CAD build for the part. Positions are in the model's coordinates, mm. Round coordinates to 2 decimals unless told otherwise and drop trailing zeros. Loops run counter-clockwise (first coordinate to the right, second up) from the corner with the lowest first, then second, coordinate; pieces in that order, holes last.
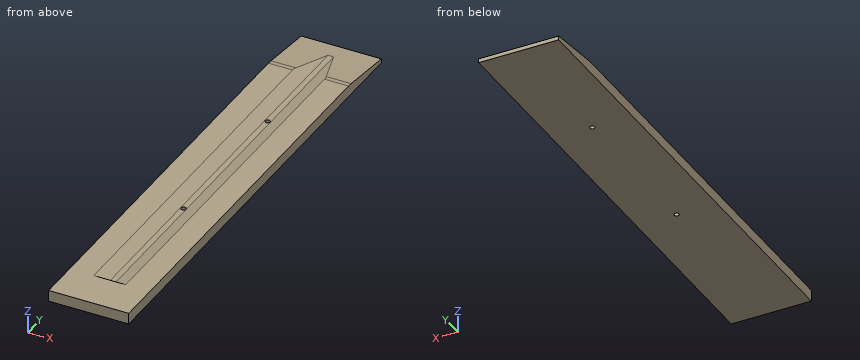
```python
from build123d import *

# Parameters (mm, degrees)
F1_DEPTH = 20
F3_DEPTH = 120
F6_R     = 0.6
F7_DEPTH = 25
F8_R     = 10


with BuildPart() as f1:
    # F0 (on Right) → F1 (new body)
    with BuildSketch(Plane.YZ):
        Polygon((0, 2.8), (0, 0), (120, 0), (120, 1), (105, 2.8), align=None)
    extrude(amount=F1_DEPTH)


with BuildPart() as f3:
    # F2 (on face) → F3 (new body)
    with BuildSketch(Plane.XZ):
        Polygon((6, 2.8), (9.296973, 1.6), (10.703027, 1.6), (14, 2.8), align=None)
    extrude(amount=-F3_DEPTH)


with BuildPart() as f3_1:
    # F4: moved
    add(f3.part.moved(Location((0, 10, 0))))


with BuildPart() as f1_1:
    add(f1.part)

    # F5: cut F3
    add(f3_1.part, mode=Mode.SUBTRACT)

    # F6 (on face) → F7 (cut)
    with BuildSketch(Plane.XY.offset(1.6)):
        with Locations((10, 85)):
            Circle(F6_R)
        with Locations((10, 45)):
            Circle(F6_R)
    extrude(amount=-F7_DEPTH, mode=Mode.SUBTRACT)

    # F8
    f8_edges = [f1_1.edges().sort_by_distance(p)[0] for p in [
        (17, 105, 2.8),
        (3, 105, 2.8),
    ]]
    fillet(f8_edges, radius=F8_R)


solid = f1_1.part
```
Item 1: Probe line 1 (Y direction, x = 10, z = 0.4); line 2 (X direction, y = 85, z = 1); line 3 (Z direction, x = 10.25, y = 96.5). List the from-to ranges inside material, lowest first.
Answers follow:
line 1: y = 0 to 44.4, 45.6 to 84.4, 85.6 to 120
line 2: x = 0 to 9.4, 10.6 to 20
line 3: z = 0 to 1.6
Item 2: Cut at C-C, the plane z = 2.15. Give the cut face in (x, y), plus the area to 3 significant figures.
Answers follow:
outline: (0, 0) - (20, 0) - (20, 110.42) - (12.21, 110.42) - (12.21, 10) - (7.79, 10) - (7.79, 110.42) - (0, 110.42) - close
area: 1,760 mm2
Item 3: Cut at A-A, the plane y = 94. Give the cut face in (x, z), plus the area to 3 significant figures.
Answers follow:
outline: (0, 0) - (20, 0) - (20, 2.8) - (14, 2.8) - (10.7, 1.6) - (9.3, 1.6) - (6, 2.8) - (0, 2.8) - close
area: 50.4 mm2
Item 4: Cut at B-B, the plane x = 15.5. Give the cut face in (y, z).
Answers follow:
outline: (0, 0) - (120, 0) - (120, 1) - (105.59, 2.73) arc R10 ccw to (104.4, 2.8) - (0, 2.8) - close
Item 5: Flat gauge pins, fed straight in: P1, Ø1.5, axis at x = 10.5, y = 46.5, coming from the +Z side; P2, Ø12, axis at x = 14, y = 100, coming from the -Z side. Where does each tip first touch, or does it go through?
Answers follow:
P1: stops at z = 1.8
P2: stops at z = 0
Item 6: Cut at D-D, the plane x = 8.25. Give the cut face in (y, z), plus the area to 3 significant figures.
Answers follow:
outline: (0, 0) - (120, 0) - (120, 1) - (111.82, 1.98) - (10, 1.98) - (10, 2.8) - (0, 2.8) - close
area: 242 mm2
